Design review of the part built by this model. Coordinates are the model's own, in mm. Face numbers are marked on the shaded views. A direction names the side the tool comes from. Coordinates: 2 decimals unless noted, no trailing zeros. Loops run counter-clockwise (first coordinate to the right, second up) from the corner with the lowest first, then second, coordinate; pieces in that order, holes last. Notation, with made-up numbers: (33.5, -3) -> (50.5, -3) arc R22 ccw to (50.5, 30) -> close; hole circle Ø10 at (-15.75, -23.5). An arc over 180 degrees is marked (long way). Use CSV: the item, a comma, the result in double quotes.
```python
from build123d import *

# Parameters (mm, degrees)
SKETCH048_R  = 17.5
PAD032_DEPTH = 10
PAD033_DEPTH = 5
FILLET011_R  = 0.5
FILLET012_R  = 0.5
FILLET013_R  = 2


with BuildPart() as part:
    # Sketch048 (on DatumPlane) → Pad032 (new body)
    with BuildSketch(Plane(origin=(0, 15.789559, -564.544271), x_dir=(0, 1, 0), z_dir=(0, 0, 1))):
        Circle(SKETCH048_R)
    extrude(amount=PAD032_DEPTH)

    # Sketch049 (on Face3 of Pad032) → Pad033 (join)
    with BuildSketch(Plane(origin=(0, 15.789559, -554.544271), x_dir=(0, 1, 0), z_dir=(0, 0, 1))):
        with BuildLine():
            ThreePointArc((-12.797492, 3.946719), (-16.744211, 0), (-12.797492, -3.946719))
            Line((-12.797492, -3.946719), (12.797492, -3.946719))
            ThreePointArc((12.797492, -3.946719), (16.744211, 0), (12.797492, 3.946719))
            Line((-12.797492, 3.946719), (12.797492, 3.946719))
        make_face()
    extrude(amount=PAD033_DEPTH)

    # Fillet011
    fillet011_edges = [part.edges().sort_by_distance(p)[0] for p in [
        (0, -1.710441, -554.544271),
    ]]
    fillet(fillet011_edges, radius=FILLET011_R)

    # Fillet012
    fillet012_edges = [part.edges().sort_by_distance(p)[0] for p in [
        (-3.946719, 15.789559, -554.544271),
    ]]
    fillet(fillet012_edges, radius=FILLET012_R)

    # Fillet013
    fillet013_edges = [part.edges().sort_by_distance(p)[0] for p in [
        (0, 32.53377, -549.544271),
    ]]
    fillet(fillet013_edges, radius=FILLET013_R)


solid = part.part
```
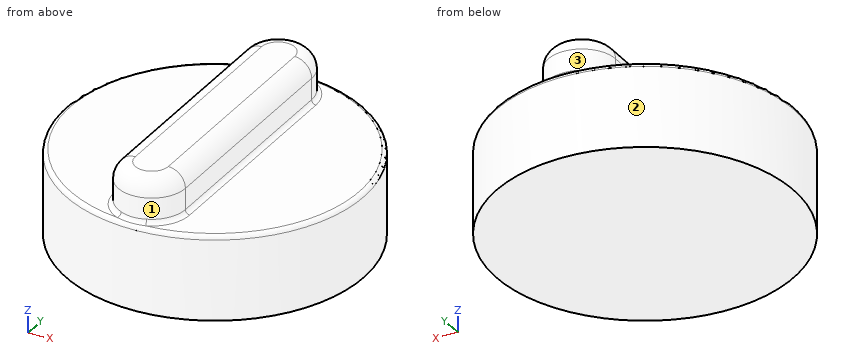
Item 1: Add section A-A (z = -559.75). Give the boundary of the cut face in (x, y).
Checked values:
outline,"circle Ø35 at (0, 15.79)"
Item 2: To check wall thickness, follow line 1 along Z through (x, y) = (4.5, 16); line 2 along X through (y, z) = (6.5, -552); line 3 along X through (y, z) = (26.5, -556.5). State the ranges of each line that lie inside material, in increasing order.
Checked values:
line 1,"-564.54 to -554.54"
line 2,"-3.95 to 3.95"
line 3,"-13.84 to 13.84"
Item 3: Machinability: for the marked faces 1, 2 and 3, which of the approach directions +Z, -Z, +X, -X, +Y, -Y give a long, thin tool a straight path to every point of the face, cutting with its end or side? Answer none if there is none.
Checked values:
face 1,"+Z, -Y"
face 2,"+Z, -Z"
face 3,"+Z, +Y"
Item 4: Clearance check with flat-ended pins moving along their axes: pin 1 (5 mm diameter, centred on y = 12, z = -563, fed in from +X); pin 2 (2 mm diameter, centred on y = 12.5, z = -552.5, fed in from +X); pin 3 (5 mm diameter, centred on x = 5, z = -561.5, fed in from -Y). State where each tip first meets the part, or that it passes through.
Checked values:
pin 1,"x = 17.45"
pin 2,"x = 3.95"
pin 3,"y = -1.53"
